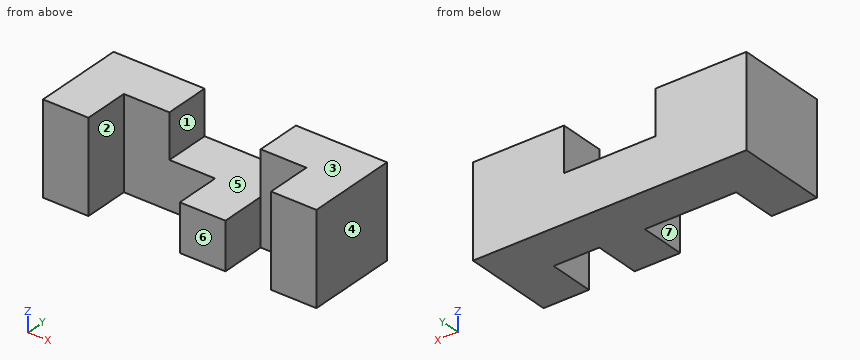
```python
from build123d import *

# Parameters (mm, degrees)
F0_W     = 76.2
F0_H     = 25.4
F1_DEPTH = 25.4
F2_W     = 25.4508
F2_H     = 12.7254
F3_DEPTH = 25.4
F4_W     = 12.7254
F4_H     = 12.7254
F5_DEPTH = 25.4
F6_W     = 25.4508
F6_H     = 12.7254
F7_DEPTH = 25.654


with BuildPart() as f1:
    # F0 (on Top) → F1 (new body)
    with BuildSketch(Plane.XY):
        with Locations((38.1, 12.7)):
            Rectangle(F0_W, F0_H)
    extrude(amount=F1_DEPTH)

    # F2 (on Front) → F3 (cut)
    with BuildSketch(Plane.XZ):
        with Locations((38.1, 19.458432)):
            Rectangle(F2_W, F2_H)
    extrude(amount=-F3_DEPTH, mode=Mode.SUBTRACT)

    # F4 (on face) → F5 (cut)
    with BuildSketch(Plane.XY.offset(25.4)):
        with Locations((57.1881, 6.3627)):
            Rectangle(F4_W, F4_H)
    extrude(amount=-F5_DEPTH, mode=Mode.SUBTRACT)

    # F6 (on Top) → F7 (cut)
    with BuildSketch(Plane.XY):
        with Locations((25.4, 6.3627)):
            Rectangle(F6_W, F6_H)
    extrude(amount=F7_DEPTH, mode=Mode.SUBTRACT)


solid = f1.part
```
Model file for the job. Use its own axes, mm. Face numbers are marked on the shaded views. A direction names the side the tool comes from. Coordinates: 2 decimals unless noted, no trailing zeros. Loops run counter-clockwise (first coordinate to the right, second up) from the corner with the lowest first, then second, coordinate; pieces in that order, holes last. Notation, with made-up numbers: M 67,47.5 L 121,47.5 A20 ccw 121,62.5 Z; hole C 6.25,8.5 d5. An arc over 180 degrees is marked long. Use CSV: the item, a comma, the result in double quotes. Start each with the question number.
1. Probe probe 1 along X at (y, z) = (7, 12.25); probe 2 along X at (y, z) = (22, 20); probe 3 along X at (y, z) = (6, 19.5). List the from-to ranges inside material, lowest first. Write a range as [from, to].
2. Band-saw the part on A-A, the plane y = 2.25. List the corners of the cut face in (x, z), then the cut area to 3 significant figures.
3. Flat gauge pins, fed straight in: pin 1 (12.5 mm diameter, centred on x = 19.5, z = 17, fed in from -Y); pin 2 (12.5 mm diameter, centred on x = 39.5, y = 6.5, fed in from +Z). Where does each tip first touch, or does it go through?
4. Two-plate mould, pull along X, no slides. Class the marked faces 4, 5, 6 and 7: pulls with the +X half, pulls with the -X half, needs draft (parallel to the pull), parting line crosses it, or undercut.
5. Band-saw the part on D-D, the plane y = 21. List the corners of the cut face in (x, z).
6. Tool access for the marked faces 1, 2 and 3: list every direction of +Z, -Z, +X, -X, +Y, -Y with a clear straight run to the whole face (end or side of a thin tool).
7. Band-saw the part on C-C, the plane z = 1.5. List the corners of the cut face in (x, y).
8. Band-saw the part on B-B, the plane z = 20.25. List the corners of the cut face in (x, y).
Entries:
1,probe 1,"x = [0, 12.67], [38.13, 50.83], [63.55, 76.2]"
1,probe 2,"x = [0, 25.37], [50.83, 76.2]"
1,probe 3,"x = [0, 12.67], [63.55, 76.2]"
2,outline,"M 0,0 L 12.67,0 L 12.67,25.4 L 0,25.4 Z; M 38.13,0 L 50.83,0 L 50.83,13.1 L 38.13,13.1 Z; M 63.55,0 L 76.2,0 L 76.2,25.4 L 63.55,25.4 Z"
2,area,"810 mm2"
3,pin 1,"stops at y = 12.73"
3,pin 2,"stops at z = 13.1"
4,face 4,"pulls with the +X half"
4,face 5,"undercut"
4,face 6,"needs draft"
4,face 7,"undercut"
5,outline,"M 0,0 L 76.2,0 L 76.2,25.4 L 50.83,25.4 L 50.83,13.1 L 25.37,13.1 L 25.37,25.4 L 0,25.4 Z"
6,face 1,"+Z, +Y, -Y"
6,face 2,"+Z, -Z, -Y"
6,face 3,"+Z, +X, -X, +Y, -Y"
7,outline,"M 0,0 L 12.67,0 L 12.67,12.73 L 38.13,12.73 L 38.13,0 L 50.83,0 L 50.83,12.73 L 63.55,12.73 L 63.55,0 L 76.2,0 L 76.2,25.4 L 0,25.4 Z"
8,outline,"M 0,0 L 12.67,0 L 12.67,12.73 L 25.37,12.73 L 25.37,25.4 L 0,25.4 Z; M 50.83,12.73 L 63.55,12.73 L 63.55,0 L 76.2,0 L 76.2,25.4 L 50.83,25.4 Z"
